Source: CAD feature listing. Evaluate the final solid. Frame: model axes, mm. Face numbers are marked on the shaded views. Give positions to 0.01 mm unless a question says otherwise; leave off trailing zeros. Loops run counter-clockwise (first coordinate to the right, second up) from the corner with the lowest first, then second, coordinate; pieces in that order, holes last.
from build123d import *

# Parameters (mm, degrees)
SKETCH1_W           = 20
SKETCH1_H           = 30
BOSS_EXTRUDE1_DEPTH = 3
SKETCH2_R           = 2.3
CUT_EXTRUDE1_DEPTH  = 3
FILLET1_R           = 3


with BuildPart() as part:
    # Sketch1 → Boss-Extrude1 (new body)
    with BuildSketch(Plane.XY):
        Rectangle(SKETCH1_W, SKETCH1_H)
    extrude(amount=BOSS_EXTRUDE1_DEPTH)

    # Sketch2 → Cut-Extrude1 (cut)
    with BuildSketch(Plane.XY.offset(3)):
        with Locations((-5.05, 10)):
            Circle(SKETCH2_R)
        with Locations((5.05, 10)):
            Circle(SKETCH2_R)
        with Locations((-5.05, -10)):
            Circle(SKETCH2_R)
        with Locations((5.05, -10)):
            Circle(SKETCH2_R)
    extrude(amount=-CUT_EXTRUDE1_DEPTH, mode=Mode.SUBTRACT)

    # Fillet1
    fillet1_edges = [part.edges().sort_by_distance(p)[0] for p in [
        (10, -15, 1.5),
        (-10, -15, 1.5),
        (-10, 15, 1.5),
        (10, 15, 1.5),
    ]]
    fillet(fillet1_edges, radius=FILLET1_R)


solid = part.part
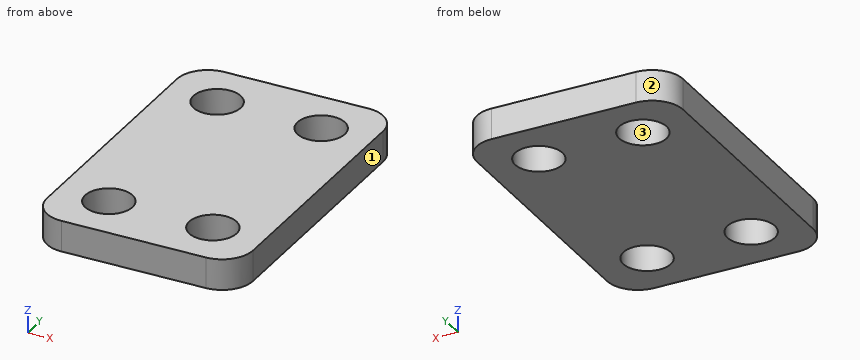
1) Cut plane D-D (x = -8.25). Return loops of the section in (y, z).
Checks:
outline: (-14.73, 0) - (14.73, 0) - (14.73, 3) - (-14.73, 3) - close
2) Cut plane B-B (z = 0.65). Return loops of the section in (x, y).
Checks:
outline: (-10, -12) arc R3 ccw to (-7, -15) - (7, -15) arc R3 ccw to (10, -12) - (10, 12) arc R3 ccw to (7, 15) - (-7, 15) arc R3 ccw to (-10, 12) - close; hole circle Ø4.6 at (-5.05, -10); hole circle Ø4.6 at (-5.05, 10); hole circle Ø4.6 at (5.05, -10); hole circle Ø4.6 at (5.05, 10)
3) Contact query for a flat-ended pin moving along its axis: P1, Ø3, axis at x = -5.05, y = -10, coming from the -Z side. Output: stop coordinate, or through.
Checks:
P1: passes through
4) Pull-direction query (X, two-part tool) for the marked faces 1, 2 and 3; classes: released by +X, released by -X, zero draft, split by the parting line, or undercut.
Checks:
face 1: released by +X
face 2: released by -X
face 3: undercut
5) Cut plane A-A (x = 5.05). Return loops of the section in (y, z).
Checks:
outline: (-15, 0) - (-12.3, 0) - (-12.3, 3) - (-15, 3) - close; (-7.7, 0) - (7.7, 0) - (7.7, 3) - (-7.7, 3) - close; (12.3, 0) - (15, 0) - (15, 3) - (12.3, 3) - close
6) Ray query, probe 1 along Y at (x, z) = (5, 1.1); probe 2 along X at (y, z) = (-12, 0.95); probe 3 along Y at (x, z) = (6, 1.8). Return the intervals inside material, ascending.
Checks:
probe 1: y = -15 to -12.3, -7.7 to 7.7, 12.3 to 15
probe 2: x = -10 to -6.19, -3.91 to 3.91, 6.19 to 10
probe 3: y = -15 to -12.09, -7.91 to 7.91, 12.09 to 15
7) Cut plane C-C (y = 10). Return loops of the section in (x, z), and give its area (3 significant figures).
Checks:
outline: (-10, 0) - (-7.35, 0) - (-7.35, 3) - (-10, 3) - close; (-2.75, 0) - (2.75, 0) - (2.75, 3) - (-2.75, 3) - close; (7.35, 0) - (10, 0) - (10, 3) - (7.35, 3) - close
area: 32.4 mm2
